from build123d import *

# Parameters (mm, degrees)
SKETCH1_W           = 61
SKETCH1_H           = 62
SKETCH1_R           = 2.675
BASE_DEPTH          = 6.45
SKETCH2_W           = 49.185
SKETCH2_H           = 62
SEMICONDUCTOR_DEPTH = 12.22
SKETCH3_W           = 11.815
SKETCH3_H           = 16.5
SKETCH3_W_2         = 11.5
SKETCH3_R           = 3.15
TABS_DEPTH          = 18.67


with BuildPart() as part:
    # Sketch1 → Base (new body)
    with BuildSketch(Plane(origin=(0, 0, 0), x_dir=(1, 0, 0), z_dir=(0, 1, 0))):
        with Locations((-30.5, 0)):
            Rectangle(SKETCH1_W, SKETCH1_H)
        with Locations((-55.095, -25.095)):
            Circle(SKETCH1_R, mode=Mode.SUBTRACT)
        with Locations((-55.095, 25.09)):
            Circle(SKETCH1_R, mode=Mode.SUBTRACT)
    extrude(amount=BASE_DEPTH)

    # Sketch2 → Semiconductor (add)
    with BuildSketch(Plane(origin=(0, 6.45, 0), x_dir=(1, 0, 0), z_dir=(0, 1, 0))):
        with Locations((-24.5925, 0)):
            Rectangle(SKETCH2_W, SKETCH2_H)
    extrude(amount=SEMICONDUCTOR_DEPTH)

    # Sketch3 → Tabs (add)
    with BuildSketch(Plane.XZ):
        with Locations((-55.0925, 11)):
            Rectangle(SKETCH3_W, SKETCH3_H)
        with Locations((-55.0925, -11)):
            Rectangle(SKETCH3_W, SKETCH3_H)
        with Locations((-66.75, -11)):
            Rectangle(SKETCH3_W_2, SKETCH3_H)
        with Locations((-65.5, -11)):
            Circle(SKETCH3_R, mode=Mode.SUBTRACT)
        with Locations((-66.75, 11)):
            Rectangle(SKETCH3_W_2, SKETCH3_H)
        with Locations((-65.5, 11)):
            Circle(SKETCH3_R, mode=Mode.SUBTRACT)
    extrude(amount=-TABS_DEPTH)

    # Mirror 2: part across plane


with BuildPart() as part_1:
    add(part.part)
    add(part.part.mirror(Plane(origin=(0, 6.45, 0), x_dir=(0, 0, 1), z_dir=(1, 0, 0))))


solid = part_1.part
Verification items for the finished model (mm, model axes). A direction names the side the tool comes from. Give positions to 0.01 mm unless a question says otherwise; leave off trailing zeros. Order: outer loops, then holes, each group sorted by start corner. A loop starts at its lowest first (then second) coordinate and runs counter-clockwise, first axis right, second up. Notation, with made-up numbers: M 16.5,-18 L 58.5,-18 A21 ccw 58.5,7 Z; hole C 47.5,-6.5 d3. An arc over 180 degrees is marked long. Answer as a JSON object with one key per item and string values. Group by question number.
1) Cross-section at A-A (x = -65.5). Enter the section's corners in (y, z).
2) Mould release check, pull along X, two halves, no side actions. Record for faces 6 (the face through (-55.7, 3.2, 27.7)), 7 (the face through (72.5, 9, -11)), 8 (the face through (-58, 6.45, 25)): released by +X, released by -X, zero draft, split by the parting line, or undercut.
3) Cross-section at C-C (z = -11). Enter the section's corners in (x, y).
4) Scan lines: line 1 along Z through (x, y) = (-65.5, 10.5); line 2 along X through (y, z) = (3.5, -25.09); line 3 along X through (y, z) = (2.25, 10). Record each from-to range of solid material in increasing order. Write a range as [from, to].
5) Cross-section at B-B (y = 8). Enter the section's corners in (x, z) (3 decimals), then the cut area to 3 significant figures.
6) Access from +Z, -Z, +X, -X, +Y, -Y to the whole of each face (thin tool, end or side, straight path). Record for faces 1 (the face through (61, 3, 0)), 2 (the face through (-49.185, 12, 25)), 3 (the face through (61, 11, -2.75)), 4 (the face through (-49.185, 12, 0)), 5 (the face through (49.185, 12, 25)).
7) Depth check by flat-ended pin: pin 1 Ø5.5 at (x, y) = (57, 11) entering from +Z; pin 2 Ø4.5 at (x, z) = (-52, 0) entering from +Y; pin 3 Ø6 at (y, z) = (14.5, -22.5) entering from -X (3 decimals). Enter the tip coordinate at first touch or a pass-through.
Result sheet:
{
 "1": {"outline": "M 0,-19.25 L 18.67,-19.25 L 18.67,-14.15 L 0,-14.15 Z; M 0,-7.85 L 18.67,-7.85 L 18.67,-2.75 L 0,-2.75 Z; M 0,2.75 L 18.67,2.75 L 18.67,7.85 L 0,7.85 Z; M 0,14.15 L 18.67,14.15 L 18.67,19.25 L 0,19.25 Z"},
 "2": {"face 6": "undercut", "face 7": "released by +X", "face 8": "zero draft"},
 "3": {"outline": "M -72.5,0 L -68.65,0 L -68.65,18.67 L -72.5,18.67 Z; M -62.35,0 L 62.35,0 L 62.35,18.67 L -62.35,18.67 Z; M 68.65,0 L 72.5,0 L 72.5,18.67 L 68.65,18.67 Z"},
 "4": {"line 1": "z = [-19.25, -14.15], [-7.85, -2.75], [2.75, 7.85], [14.15, 19.25]", "line 2": "x = [-61, -57.77], [-52.42, 52.42], [57.77, 61]", "line 3": "x = [-72.5, -68.49], [-62.51, 62.51], [68.49, 72.5]"},
 "5": {"outline": "M -72.5,-19.25 L -49.185,-19.25 L -49.185,-31 L 49.185,-31 L 49.185,-19.25 L 72.5,-19.25 L 72.5,-2.75 L 49.185,-2.75 L 49.185,2.75 L 72.5,2.75 L 72.5,19.25 L 49.185,19.25 L 49.185,31 L -49.185,31 L -49.185,19.25 L -72.5,19.25 L -72.5,2.75 L -49.185,2.75 L -49.185,-2.75 L -72.5,-2.75 Z; hole C -65.5,-11 d6.3; hole C -65.5,11 d6.3; hole C 65.5,-11 d6.3; hole C 65.5,11 d6.3", "area": "7,510 mm2"},
 "6": {"face 1": "+X, +Y, -Y", "face 2": "+Z, -X, +Y", "face 3": "+X, +Y", "face 4": "-X, +Y", "face 5": "+Z, +X, +Y"},
 "7": {"pin 1": "stops at z = 19.25", "pin 2": "stops at y = 6.45", "pin 3": "stops at x = -49.185"}
}
